Part print with two shaded views. Sizes in mm from the minimum x, y, z corner. A direction names the side the tool comes from. Round coordinates to 2 decimals unless told otherwise and drop trailing zeros. Loops run counter-clockwise (first coordinate to the right, second up) from the corner with the lowest first, then second, coordinate; pieces in that order, holes last. Notation, with made-up numbers: M -29,78.5 L 3,78.5 A15 cw 3,97.5 Z; hole C 11.25,26 d7. An arc over 180 degrees is marked long. Use a Markdown table: item, result. Add a question column.
Item 1: Saw through at B-B on y = 2.5. Write the cut outline in (x, z).
Item 2: Saw through at A-A on x = 42. Write the cut outline in (y, z).
Item 3: Saw through at D-D on x = 25. Write the cut outline in (y, z).
Item 4: Tool access for the marked faces 4 and 5: list every direction of +Z, -Z, +X, -X, +Y, -Y with a clear straight run to the whole face (end or side of a thin tool).
Item 5: Pin check, flat tip, straight feed: P1, Ø1.5, axis at x = 13.5, z = 42.5, coming from the +Y side. Stop position of the tip, or through.
Item 6: Wall check: L1, parallel to X at y = 19.5, z = 6; L2, parallel to Y at x = 3.95, z = 25. Give the ranges that are in metal, low to high. Write a range as from..to.
Item 7: Two-plate mould, pull along Z, no slides. Class the marked faces 1, 2 and 3: +Z half, -Z half, draft (parallel to the pull), parting line (faces both ways), or undercut.
Item 8: Saw through at C-C on z = 25. Write the cut outline in (x, y).
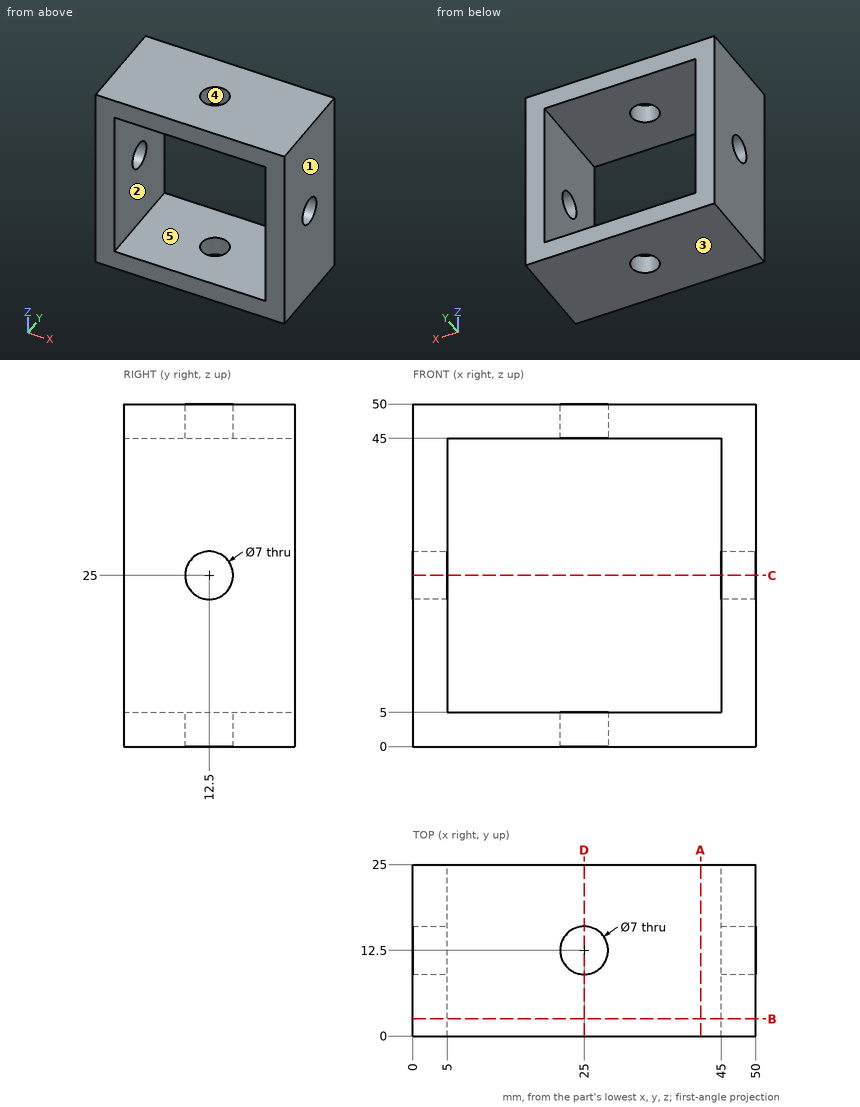
Entries:
| question | item | result |
|---|---|---|
| 1 | outline | M 0,0 L 50,0 L 50,50 L 0,50 Z; hole M 5,5 L 45,5 L 45,45 L 5,45 Z |
| 2 | outline | M 0,0 L 25,0 L 25,5 L 0,5 Z; M 0,45 L 25,45 L 25,50 L 0,50 Z |
| 3 | outline | M 0,0 L 9,0 L 9,5 L 0,5 Z; M 0,45 L 9,45 L 9,50 L 0,50 Z; M 16,0 L 25,0 L 25,5 L 16,5 Z; M 16,45 L 25,45 L 25,50 L 16,50 Z |
| 4 | face 4 | +Z, -Z |
| 4 | face 5 | +Y, -Y |
| 5 | P1 | through |
| 6 | L1 | 0..5, 45..50 |
| 6 | L2 | 0..9, 16..25 |
| 7 | face 1 | draft |
| 7 | face 2 | undercut |
| 7 | face 3 | -Z half |
| 8 | outline | M 0,0 L 5,0 L 5,9 L 0,9 Z; M 0,16 L 5,16 L 5,25 L 0,25 Z; M 45,0 L 50,0 L 50,9 L 45,9 Z; M 45,16 L 50,16 L 50,25 L 45,25 Z |
